Study the drawing (mm; zero at the part's minimum x, y, z) and answer. A direction names the side the tool comes from. Give positions to 0.01 mm unless a question says otherwise; leave off trailing zeros. Order: outer loops, then holes, each group sorted by start corner. A loop starts at its lowest first (then second) coordinate and runs counter-clockwise, first axis right, second up.
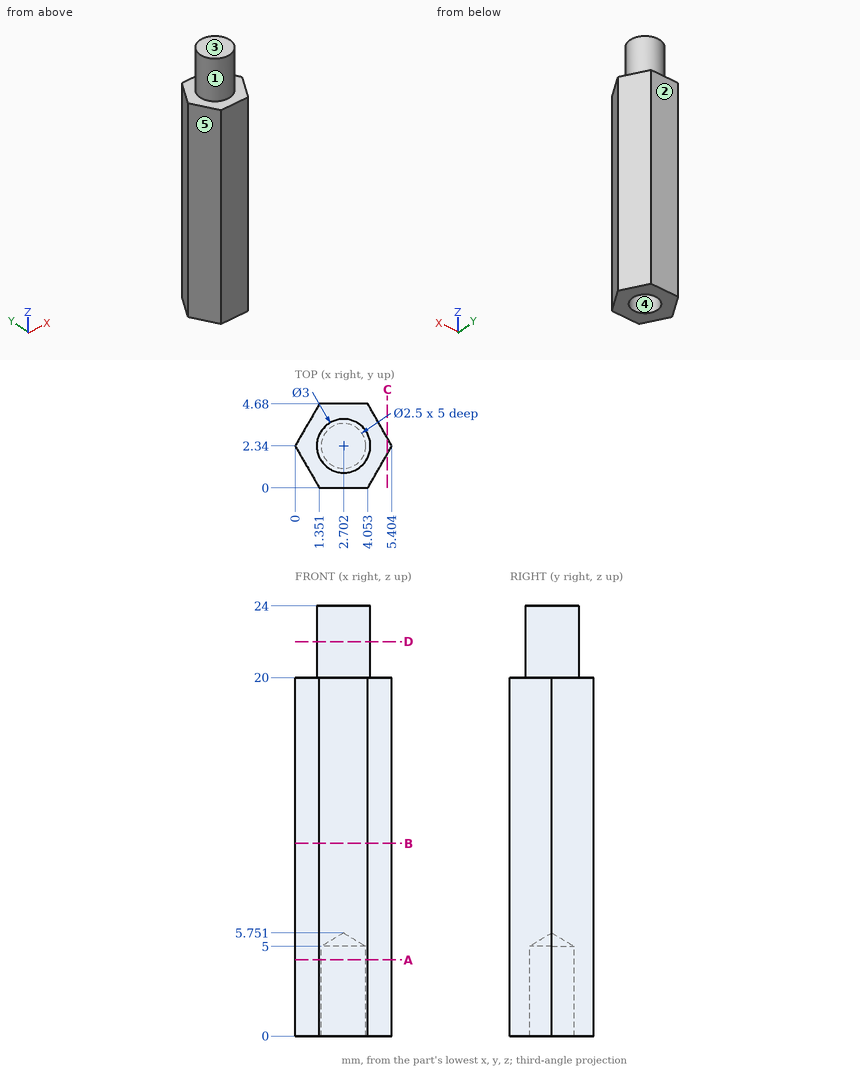
1) Find section C-C (x = 5.15). Write down the section's boundary in (y, z).
Geometry says:
outline: (1.9, 0) - (2.78, 0) - (2.78, 20) - (1.9, 20) - close
2) A tool of negligible diameter and unlimited length cuts with its end or side. For the marked faces 1 and 2, from which of +Z, -Z, +X, -X, +Y, -Y can it reach the whole face along a straight path? Write none if from no direction.
Geometry says:
face 1: +Z
face 2: +Z, -Z, +X, -X, +Y
3) Given P1, Ø1.5, axis at y = 4, z = 9.5, coming from the +X side, flat-ended and moving along its own axis, determine where the tip first touches the part or whether it passes through.
Geometry says:
P1: stops at x = 4.88
4) Straight lines are drawn through the part: probe 1 along X at (y, z) = (2.1, 3) (1 decimal); probe 2 along Z at (x, y) = (1.65, 4.25); probe 3 along X at (y, z) = (1.9, 5.75). For each, find the intervals that lie inside material, in ascending order.
Geometry says:
probe 1: x = 0.1 to 1.5, 3.9 to 5.3
probe 2: z = 0 to 20
probe 3: x = 0.25 to 5.15
5) Find section D-D (z = 22). Write down the section's boundary in (x, y), then the cut area to 3 significant figures.
Geometry says:
outline: circle Ø3 at (2.7, 2.34)
area: 7.07 mm2
6) For a pull along X with two mould halves and no side action, classify the marked faces 3, 4 and 5 as +X half, -X half, draft (parallel to the pull), parting line (faces both ways), or undercut.
Geometry says:
face 3: draft
face 4: undercut
face 5: -X half
7) Find section A-A (z = 4.25). Write down the section's boundary in (x, y).
Geometry says:
outline: (0, 2.34) - (1.35, 0) - (4.05, 0) - (5.4, 2.34) - (4.05, 4.68) - (1.35, 4.68) - close; hole circle Ø2.5 at (2.7, 2.34)
8) Find section B-B (z = 10.75). Write down the section's boundary in (x, y).
Geometry says:
outline: (0, 2.34) - (1.35, 0) - (4.05, 0) - (5.4, 2.34) - (4.05, 4.68) - (1.35, 4.68) - close
